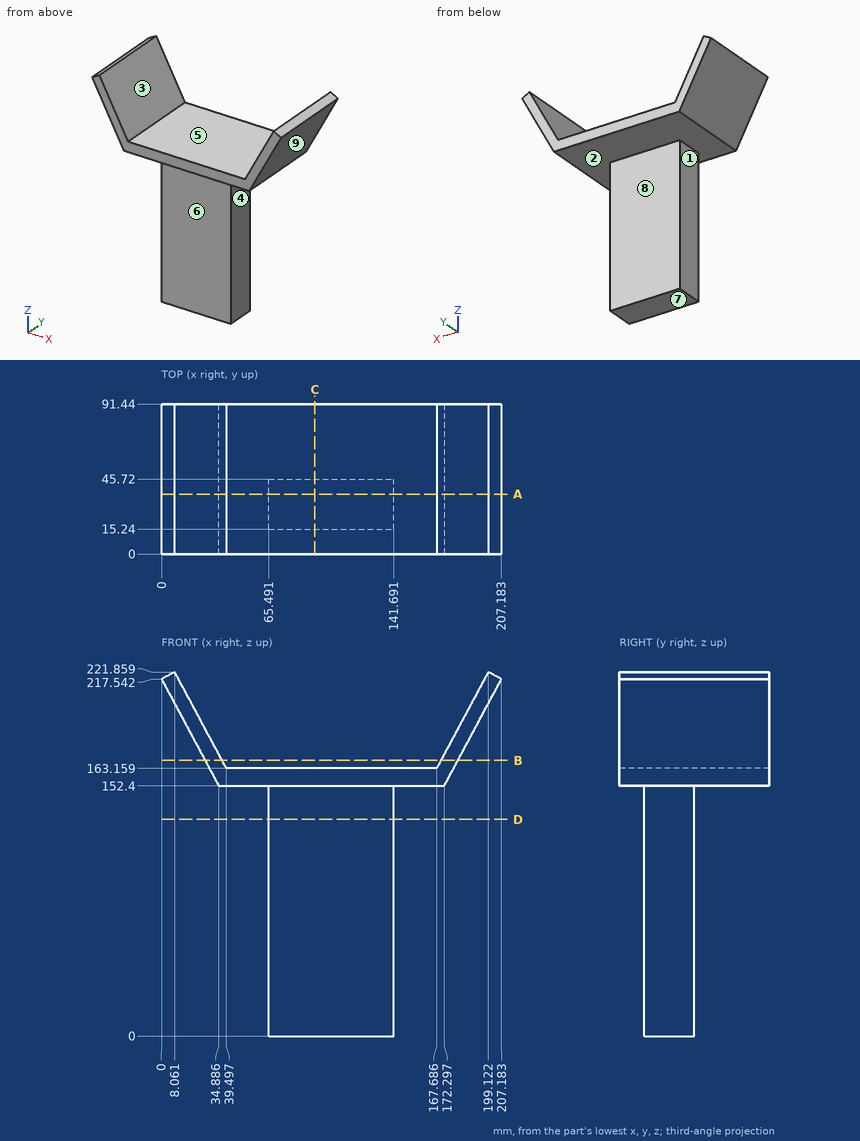
The drawing under review shows one solid part. Ordinate dimensions are in mm from its lowest x, y, z. A direction names the side the tool comes from. Coordinates: 2 decimals unless noted, no trailing zeros. Loops run counter-clockwise (first coordinate to the right, second up) from the corner with the lowest first, then second, coordinate; pieces in that order, holes last. Notation, with made-up numbers: M -30,85.25 L 28,85.25 A22 cw 28,113.25 Z; hole C 67.5,12 d10. An arc over 180 degrees is marked long. Use one line per item in the form item = value.
(1) Consider section C-C (x = 93.5). Write out the cut boundary in (y, z), and give its area (3 significant figures).
Return value:
outline = M 0,152.4 L 15.24,152.4 L 15.24,0 L 45.72,0 L 45.72,152.4 L 91.44,152.4 L 91.44,163.16 L 0,163.16 Z
area = 5,630 mm2
(2) Draft analysis for pull direction X (two halves, no side actions). For the marked faces 1, 2, 3 and 4, state which applies: pulls with the +X half, pulls with the -X half, needs draft (parallel to the pull), parting line crosses it, or undercut.
Return value:
face_1 = pulls with the -X half
face_2 = needs draft
face_3 = undercut
face_4 = pulls with the +X half
(3) For line 1 along Z through (x, y) = (103.5, 83.5); line 2 along X through (y, z) = (68, 181) (1 decimal); line 3 along Z through (x, y) = (108, 17), list the stretches that pass through material, from the lowest coordinate up. Write a range as from..to.
Return value:
line_1 = 152.4..163.16
line_2 = 19.6..29.9, 177.2..187.6
line_3 = 0..163.16
(4) Consider section A-A (y = 36.5). Write out the cut boundary in (x, z) (1 decimal).
Return value:
outline = M 0,217.5 L 34.9,152.4 L 65.5,152.4 L 65.5,0 L 141.7,0 L 141.7,152.4 L 172.3,152.4 L 207.2,217.5 L 199.1,221.9 L 167.7,163.2 L 39.5,163.2 L 8.1,221.9 Z
(5) For the marked faces 5, 6, 7, 8 and 9, list the 3-axis set-ups (+Z, -Z, +X, -X, +Y, -Y) from which the entire face can be reached by the end or side of a thin tool; tool diameter is ignored.
Return value:
face_5 = +Z, +Y, -Y
face_6 = -Z, +X, -X, -Y
face_7 = -Z, +X, -X, +Y, -Y
face_8 = -Z, +X, -X, +Y
face_9 = -Z, +X, +Y, -Y
(6) Consider section B-B (z = 168). Write out the cut boundary in (x, y) (1 decimal).
Return value:
outline = M 26.5,0 L 36.9,0 L 36.9,91.4 L 26.5,91.4 Z; M 170.3,0 L 180.7,0 L 180.7,91.4 L 170.3,91.4 Z
(7) Consider section D-D (z = 132). Write out the cut boundary in (x, y), and give its area (3 significant figures).
Return value:
outline = M 65.49,15.24 L 141.69,15.24 L 141.69,45.72 L 65.49,45.72 Z
area = 2,320 mm2
(8) Clearance check with flat-ended pins moving along their axes: P1, Ø1, axis at y = 30.5, z = 156.5, coming from the -X side; P2, Ø6, axis at x = 60, z = 131.5, coming from the -Y side; P3, Ø1.5, axis at y = 18.5, z = 152.5, coming from the +X side; P4, Ø10, axis at y = 17, z = 52, coming from the +X side. State where each tip first meets the part, or that it passes through.
Return value:
P1 = 32.42
P2 = through
P3 = 172.75
P4 = 141.69
